from build123d import *

# Parameters (mm, degrees)
F0_R     = 1.5
F0_R_2   = 4
F0_R_3   = 30
F0_R_4   = 15
F1_DEPTH = 3


with BuildPart() as f1:
    # F0 (on Front) → F1 (new body)
    with BuildSketch(Plane.XZ):
        Polygon((-100, -20.833333), (-100, -62.5), (-33.333333, -62.5), (-33.333333, -59.5), (33.333333, -59.5), (33.333333, -62.5), (100, -62.5), (100, -20.833333), (97, -20.833333), (97, 20.833333), (100, 20.833333), (100, 62.5), (33.333333, 62.5), (33.333333, 59.5), (-33.333333, 59.5), (-33.333333, 62.5), (-100, 62.5), (-100, 20.833333), (-97, 20.833333), (-97, -20.833333), align=None)
        with Locations((-67, -25.131546)):
            Circle(F0_R, mode=Mode.SUBTRACT)
        with Locations((-13, -25.131546)):
            Circle(F0_R, mode=Mode.SUBTRACT)
        with Locations((0, -52.2)):
            Circle(F0_R, mode=Mode.SUBTRACT)
        with Locations((40, -35)):
            Circle(F0_R_2, mode=Mode.SUBTRACT)
        with Locations((-89.7, 0)):
            Circle(F0_R, mode=Mode.SUBTRACT)
        with Locations((-67, 28.868454)):
            Circle(F0_R, mode=Mode.SUBTRACT)
        with Locations((-40, 0)):
            Circle(F0_R_3, mode=Mode.SUBTRACT)
        with Locations((-13, 28.868454)):
            Circle(F0_R, mode=Mode.SUBTRACT)
        with Locations((15.5, 0)):
            Circle(F0_R, mode=Mode.SUBTRACT)
        with Locations((40, 0)):
            Circle(F0_R_4, mode=Mode.SUBTRACT)
        with Locations((64.5, 0)):
            Circle(F0_R, mode=Mode.SUBTRACT)
        with Locations((89.7, 0)):
            Circle(F0_R, mode=Mode.SUBTRACT)
        with Locations((0, 52.2)):
            Circle(F0_R, mode=Mode.SUBTRACT)
    extrude(amount=F1_DEPTH)


with BuildPart() as f2_1:
    # F2: copy of F1
    add(f1.part.moved(Location((0, 60, 0))))


solid = f1.part
Input: part model. Units: mm. Frame: model coordinates. Coordinates: 2 decimals unless noted, no trailing zeros. Loops run counter-clockwise (first coordinate to the right, second up) from the corner with the lowest first, then second, coordinate; pieces in that order, holes last. Notation, with made-up numbers: (12, 14.5) - (42, 14.5) arc R21 ccw to (42, 30.5) - close; hole circle Ø6 at (60, -30). An arc over 180 degrees is marked (long way). Answer in a Markdown table with one row per item. Add a question column.
Item 1: Line query: line 1 along Z through (x, y) = (0, -1.9); line 2 along Z through (x, y) = (64.5, -1.1); line 3 along X through (y, z) = (-2.5, -8.5). Output: solid intervals per line, ascending. Write a range as [from, to].
Item 2: Contact query for flat-ended pins moving along their axis: P1, Ø1.8, axis at x = -13, z = 28.87, coming from the +Y side; P2, Ø1.5, axis at x = -8.5, y = -1, coming from the -Z side; P3, Ø0.9, axis at y = -1, z = 8, coming from the -X side. Output: stop coordinate, or through.
Item 3: Mould query, pull axis Z, two halves, no side actions, for faces 1 (the cylindrical face through (-62.111, -1.479, 20.275)), 2 (the flat face through (-1, -3, 1)). Classes: released by +Z, released by -Z, zero draft, split by the parting line, or undercut.
Item 4: Section query B-B on z = -18. Return the cut outline in (x, y), then the cut area to 3 significant figures.
Item 5: Section query C-C on y = -2.35. State how many separate pieces and enclosed holes the cut face has, then the cut area to 3 significant figures.
Item 6: Section query A-A on x = -40. Return the cut outline in (y, z), then the cut area to 3 significant figures.
Recorded:
| question | item | result |
|---|---|---|
| 1 | line 1 | [-59.5, -53.7], [-50.7, 50.7], [53.7, 59.5] |
| 1 | line 2 | [-62.5, -1.5], [1.5, 62.5] |
| 1 | line 3 | [-97, -68.77], [-11.23, 27.64], [52.36, 97] |
| 2 | P1 | through |
| 2 | P2 | z = -59.5 |
| 2 | P3 | x = -97 |
| 3 | face 1 | undercut |
| 3 | face 2 | zero draft |
| 4 | outline | (-97, -3) - (-64, -3) - (-64, 0) - (-97, 0) - close; (-16, -3) - (97, -3) - (97, 0) - (-16, 0) - close |
| 4 | area | 438 mm^2 |
| 5 | separate pieces | 1 |
| 5 | enclosed holes | 13 |
| 5 | area | 20,700 mm^2 |
| 6 | outline | (-3, -62.5) - (0, -62.5) - (0, -30) - (-3, -30) - close; (-3, 30) - (0, 30) - (0, 62.5) - (-3, 62.5) - close |
| 6 | area | 195 mm^2 |
